```python
from build123d import *

# Parameters (mm, degrees)
F0_W      = 40
F0_H      = 72
F0_W_2    = 35
F0_H_2    = 67
F1_DEPTH  = 20
F0_W_3    = 50
F0_H_3    = 82
F2_DEPTH  = 2
F3_DEPTH  = 18
F4_W      = 14
F4_H      = 7.8402353459
F5_DEPTH  = 5
F6_W      = 30
F6_H      = 10
F7_DEPTH  = 5
F8_W      = 34
F8_H      = 13
F9_DEPTH  = 126.25
F10_W     = 5
F10_H     = 5.1396135241
F10_W_2   = 33.6195547134
F10_H_2   = 5
F10_H_3   = 4.6385318637
F10_W_3   = 6.1518945545
F11_DEPTH = 5


with BuildPart() as f1:
    # F0 (on Top) → F1 (new body)
    with BuildSketch(Plane.XY):
        Rectangle(F0_W, F0_H)
        Rectangle(F0_W_2, F0_H_2, mode=Mode.SUBTRACT)
        Rectangle(F0_W_2, F0_H_2)
    extrude(amount=-F1_DEPTH)

    # F0 (on Top) → F2 (join)
    with BuildSketch(Plane.XY):
        Rectangle(F0_W_3, F0_H_3)
        Rectangle(F0_W, F0_H, mode=Mode.SUBTRACT)
    extrude(amount=-F2_DEPTH)

    # F0 (on Top) → F3 (cut)
    with BuildSketch(Plane.XY):
        Rectangle(F0_W_2, F0_H_2)
    extrude(amount=-F3_DEPTH, mode=Mode.SUBTRACT)

    # F4 (on face) → F5 (cut)
    with BuildSketch(Plane.YZ.offset(20)):
        with Locations((23, -5.920117673)):
            Rectangle(F4_W, F4_H)
    extrude(amount=-F5_DEPTH, mode=Mode.SUBTRACT)

    # F6 (on face) → F7 (cut)
    with BuildSketch(Plane(origin=(-20, 0, 0), x_dir=(0, -1, 0), z_dir=(-1, 0, 0))):
        with Locations((-11, -7)):
            Rectangle(F6_W, F6_H)
    extrude(amount=-F7_DEPTH, mode=Mode.SUBTRACT)

    # F8 (on face) → F9 (cut)
    with BuildSketch(Plane(origin=(0, 36, 0), x_dir=(-1, 0, 0), z_dir=(0, 1, 0))):
        with Locations((0, -8.5)):
            Rectangle(F8_W, F8_H)
    extrude(amount=-F9_DEPTH, mode=Mode.SUBTRACT)

    # F10 (on face) → F11 (cut)
    with BuildSketch(Plane.XY):
        with Locations((22.5, 23.4971074387)):
            Rectangle(F10_W, F10_H)
        with Locations((0.0185417011, 38.5)):
            Rectangle(F10_W_2, F10_H_2)
        with Locations((0.0185417011, 33.6807340682)):
            Rectangle(F10_W_2, F10_H_3)
        with Locations((16.9240527228, 23.4971074387)):
            Rectangle(F10_W_3, F10_H)
    extrude(amount=-F11_DEPTH, mode=Mode.SUBTRACT)


solid = f1.part
```
Design review of the part built by this model. Coordinates are the model's own, in mm. A direction names the side the tool comes from. Give positions to 0.01 mm unless a question says otherwise; leave off trailing zeros. Order: outer loops, then holes, each group sorted by start corner. A loop starts at its lowest first (then second) coordinate and runs counter-clockwise, first axis right, second up. Notation, with made-up numbers: (41.25, -10.75) -> (48.25, -10.75) arc R35 cw to (48.25, 27.25) -> close; hole circle Ø9 at (-23, 51). An arc over 180 degrees is marked (long way). Write item = value, one per line. Start each with the question number.
(1) We need section A-A on x = -13. Write out the cut boundary in (y, z).
(2) For pin 1 (4 mm diameter, centred on y = -1, z = -16, fed in from -X); pin 2 (1.5 mm diameter, centred on y = 20.5, z = -7.5, fed in from +X); pin 3 (6 mm diameter, centred on x = 7, y = 28.5, fed in from +Z); pin 4 (0.8 mm diameter, centred on y = -34.5, z = -9.5, fed in from +X), all flat-tipped, find the tip position at first contact; note any pin that passes through.
(3) For faces 1 (the face through (19, 23, -9.84)), 2 (the face through (-1, 33.5, -16)), 3 (the face through (17, -35, -9)), list the 3-axis set-ups (+Z, -Z, +X, -X, +Y, -Y) from which the entire face can be reached by the end or side of a thin tool; tool diameter is ignored.
(4) Mouldability with a two-part tool opening along Z and no side actions: class faces 4 (the face through (19, 16, -6)), 5 (the face through (-19, -4, -7)), 6 (the face through (-19, -9, 0)), 7 (the face through (21, 20.927, -1)) as +Z half, -Z half, draft (parallel to the pull), parting line (faces both ways), or undercut.
(5) We need section B-B on z = -4. Write out the cut boundary in (x, y), plus the area to 3 significant figures.
(6) To check wall thickness, follow line 1 along X through (y, z) = (-34.5, -8.25); line 2 along Y through (x, z) = (-8, -15.5); line 3 along X through (y, z) = (-12, -8.25). State the ranges of each line that lie inside material, in increasing order.
(7) We need section C-C on y = 24.5. Write out the cut boundary in (x, z).
(8) We need section D-D on z = -13.25. Write out the cut boundary in (x, y).
Numbers:
q1.outline = (-41, -2) -> (-33.5, -2) -> (-33.5, 0) -> (-41, 0) -> close; (-36, -20) -> (36, -20) -> (36, -15) -> (33.5, -15) -> (33.5, -18) -> (-33.5, -18) -> (-33.5, -15) -> (-36, -15) -> close
q2.pin_1 = -20
q2.pin_2 = through
q2.pin_3 = -18
q2.pin_4 = 20
q3.face_1 = +X
q3.face_2 = +Z
q3.face_3 = +Y, -Y
q4.face_4 = undercut
q4.face_5 = undercut
q4.face_6 = +Z half
q4.face_7 = draft
q5.outline = (-20, -36) -> (-17, -36) -> (-17, -33.5) -> (-17.5, -33.5) -> (-17.5, -4) -> (-20, -4) -> close; (-20, 26) -> (-17.5, 26) -> (-17.5, 33.5) -> (-17, 33.5) -> (-17, 36) -> (-20, 36) -> close; (17, -36) -> (20, -36) -> (20, 16) -> (17.5, 16) -> (17.5, -33.5) -> (17, -33.5) -> close; (17, 33.5) -> (17.5, 33.5) -> (17.5, 30) -> (20, 30) -> (20, 36) -> (17, 36) -> close
q5.area = 255 mm^2
q6.line_1 = -20 to -17, 17 to 20
q6.line_2 = -36 to -33.5, 33.5 to 36
q6.line_3 = -20 to -17.5, 17.5 to 20
q7.outline = (-25, -2) -> (-17.5, -2) -> (-17.5, 0) -> (-25, 0) -> close; (-20, -20) -> (20, -20) -> (20, -9.84) -> (17.5, -9.84) -> (17.5, -18) -> (-17.5, -18) -> (-17.5, -12) -> (-20, -12) -> close
q8.outline = (-20, -36) -> (-17, -36) -> (-17, -33.5) -> (-17.5, -33.5) -> (-17.5, 33.5) -> (-17, 33.5) -> (-17, 36) -> (-20, 36) -> close; (17, -36) -> (20, -36) -> (20, 36) -> (17, 36) -> (17, 33.5) -> (17.5, 33.5) -> (17.5, -33.5) -> (17, -33.5) -> close
